from build123d import *

# Parameters (mm, degrees)
SKETCH2_R           = 7.5
BOSS_EXTRUDE1_DEPTH = 5
FILLET1_R           = 1


with BuildPart() as part:
    # Sketch2 → Boss-Extrude1 (new body)
    with BuildSketch(Plane.XY):
        Circle(SKETCH2_R)
        with BuildLine():
            Line((-2, 3.156854249), (2, 3.156854249))
            Line((2, 3.156854249), (2, 5.656854249))
            ThreePointArc((2, 5.656854249), (0, -6), (-2, 5.656854249))
            Line((-2, 5.656854249), (-2, 3.156854249))
        make_face(mode=Mode.SUBTRACT)
    extrude(amount=BOSS_EXTRUDE1_DEPTH)

    # Fillet1
    fillet1_edges = [part.edges().sort_by_distance(p)[0] for p in [
        (-2, 3.156854249, 2.5),
        (2, 3.156854249, 2.5),
    ]]
    fillet(fillet1_edges, radius=FILLET1_R)


solid = part.part
Design review of the part built by this model. Coordinates are the model's own, in mm. A direction names the side the tool comes from. Give positions to 0.01 mm unless a question says otherwise; leave off trailing zeros. Loops run counter-clockwise (first coordinate to the right, second up) from the corner with the lowest first, then second, coordinate; pieces in that order, holes last. Notation, with made-up numbers: (25, 44) - (49, 44) arc R14 ccw to (49, 61) - close; hole circle Ø10 at (50.25, -36.75). An arc over 180 degrees is marked (long way). Write item = value, one per line.
1) To check wall thickness, follow line 1 (Y direction, x = 0, z = 1.85); line 2 (X direction, y = 3.25, z = 3.7); line 3 (X direction, y = 4, z = 4.3). State the ranges of each line that lie inside material, in increasing order.
Result sheet:
line_1 = -7.5 to -6, 3.16 to 7.5
line_2 = -6.76 to -5.04, -1.42 to 1.42, 5.04 to 6.76
line_3 = -6.34 to -4.47, -1.99 to 1.99, 4.47 to 6.34
2) Take a section at C-C on z = 1.9. State the section outline as (x, y) points.
Result sheet:
outline = circle Ø15 at (0, 0); hole (-2, 4.16) - (-2, 5.66) arc R6 ccw (long way) to (2, 5.66) - (2, 4.16) arc R1 cw to (1, 3.16) - (-1, 3.16) arc R1 cw to start
3) Take a section at A-A on x = 0. State the section outline as (y, z) points, and give its area (3 significant figures).
Result sheet:
outline = (-7.5, 0) - (-6, 0) - (-6, 5) - (-7.5, 5) - close; (3.16, 0) - (7.5, 0) - (7.5, 5) - (3.16, 5) - close
area = 29.2 mm2
4) Clearance check with flat-ended pins moving along their axes: pin 1 Ø3 at (x, z) = (-3, 2) entering from -Y; pin 2 Ø1 at (x, y) = (-5, 0.5) entering from +Z; pin 3 Ø1.2 at (y, z) = (5.5, 2) entering from +X; pin 4 Ø3 at (x, z) = (-2.5, 2.5) entering from -Y. State where each tip first meets the part, or that it passes through.
Result sheet:
pin_1 = -7.35
pin_2 = through
pin_3 = 5.68
pin_4 = -7.43
5) Draft analysis for pull direction X (two halves, no side actions). For faces 3 (the face through (1.715, 3.458, 2.535)), 4 (the face through (0, 3.4, 5)), 5 (the face through (-7.493, 0.33, 2.465)), state which applies: +X half, -X half, draft (parallel to the pull), parting line (faces both ways), or undercut.
Result sheet:
face_3 = undercut
face_4 = draft
face_5 = parting line
6) Take a section at B-B on y = 0. State the section outline as (x, z) points.
Result sheet:
outline = (-7.5, 0) - (-6, 0) - (-6, 5) - (-7.5, 5) - close; (6, 0) - (7.5, 0) - (7.5, 5) - (6, 5) - close
7) Tool access review of faces 1 (the face through (0, 3.4, 0)), 2 (the face through (2, 5, 2)): name each direction out of +Z, -Z, +X, -X, +Y, -Y from which nothing blocks a thin tool from reaching the whole face with its end or side.
Result sheet:
face_1 = -Z, +X, -X, +Y, -Y
face_2 = +Z, -Z
